Here's how the part is built. I have some questions about the finished solid (model axes, mm). Give positions to 0.01 mm unless a question says otherwise; leave off trailing zeros. Write each loop counter-clockwise with the first axis right and the second up, starting at its lowest first coordinate (ties: lowest second). Pieces come first, ordered by that corner, then holes. Notation, with made-up numbers: (57, 10) -> (67, 10) arc R27 cw to (67, 35) -> close; hole circle Ø1 at (-18.75, 86). An arc over 180 degrees is marked (long way). Use one line per item in the form item = value.
```python
from build123d import *

# Parameters (mm, degrees)
SKETCH1_R           = 15.875
SKETCH1_R_2         = 6.35
BOSS_EXTRUDE1_DEPTH = 9.525
SKETCH2_R           = 1.905
CUT_EXTRUDE1_DEPTH  = 9.525
CIRPATTERN1_COUNT   = 4


with BuildPart() as part:
    # Sketch1 → Boss-Extrude1 (new body)
    with BuildSketch(Plane.XY):
        Circle(SKETCH1_R)
        Circle(SKETCH1_R_2, mode=Mode.SUBTRACT)
    extrude(amount=BOSS_EXTRUDE1_DEPTH)

    # Sketch2 → Cut-Extrude1 (cut)
    with BuildSketch(Plane.XY.offset(9.525)):
        with Locations((0, 9.779)):
            Circle(SKETCH2_R)
    cut_extrude1 = extrude(amount=-CUT_EXTRUDE1_DEPTH, mode=Mode.SUBTRACT)

    # CirPattern1: Cut-Extrude1 ×4 about axis
    cirpattern1_axis = Axis((0, 0, 0), (0, 0, 1))
    for i in range(1, CIRPATTERN1_COUNT):
        add(cut_extrude1.rotate(cirpattern1_axis, i * 360 / CIRPATTERN1_COUNT), mode=Mode.SUBTRACT)


solid = part.part
```
Q1. Will these pins go through, and if not, where does the flat tip stop? pin 1 Ø1.5 at (x, z) = (-6.5, 4) entering from +Y; pin 2 Ø2 at (x, z) = (3, 1.5) entering from -Y; pin 3 Ø2 at (x, z) = (-1.5, 2.5) entering from -Y; pin 4 Ø3.5 at (x, y) = (0, -9.779) entering from +Z.
Result set:
pin_1 = 14.8
pin_2 = -15.75
pin_3 = -15.87
pin_4 = through
Q2. I want a section at C-C, the plane y = -4.5. Write out the boundary of the cut face in (x, z) (3 decimals).
Result set:
outline = (-15.224, 0) -> (-4.48, 0) -> (-4.48, 9.525) -> (-15.224, 9.525) -> close; (4.48, 0) -> (15.224, 0) -> (15.224, 9.525) -> (4.48, 9.525) -> close
Q3. I want a section at A-A, the plane y = 0. Write out the boundary of the cut face in (x, z) (3 decimals).
Result set:
outline = (-15.875, 0) -> (-11.684, 0) -> (-11.684, 9.525) -> (-15.875, 9.525) -> close; (-7.874, 0) -> (-6.35, 0) -> (-6.35, 9.525) -> (-7.874, 9.525) -> close; (6.35, 0) -> (7.874, 0) -> (7.874, 9.525) -> (6.35, 9.525) -> close; (11.684, 0) -> (15.875, 0) -> (15.875, 9.525) -> (11.684, 9.525) -> close
Q4. If I drill on line 1 along Y through (x, z) = (0, 4) (3 decimals); line 2 along X through (y, z) = (-0.5, 6.25); line 3 along X through (y, z) = (5, 0.5), over which ranges is the centre line in solid material (lowest first)? Write a range as from..to.
Result set:
line_1 = -15.875..-11.684, -7.874..-6.35, 6.35..7.874, 11.684..15.875
line_2 = -15.87..-11.62, -7.94..-6.33, 6.33..7.94, 11.62..15.87
line_3 = -15.07..-3.91, 3.91..15.07
Q5. I want a section at D-D, the plane x = 10.5. Write out the boundary of the cut face in (y, z) (3 decimals).
Result set:
outline = (-11.907, 0) -> (-1.763, 0) -> (-1.763, 9.525) -> (-11.907, 9.525) -> close; (1.763, 0) -> (11.907, 0) -> (11.907, 9.525) -> (1.763, 9.525) -> close
Q6. If we mould it in two halves opening along Y, with no side actions, what happens to faces 1 (the face through (-0.248, 11.668, 4.829)), 2 (the face through (-3.441, -15.497, 4.696)), 3 (the face through (7, 0, 9.525)), 4 (the face through (11.668, 0.248, 4.829))? For each: +Y half, -Y half, draft (parallel to the pull), parting line (faces both ways), or undercut.
Result set:
face_1 = undercut
face_2 = parting line
face_3 = draft
face_4 = undercut
